```python
from build123d import *

# Parameters (mm, degrees)
F1_DEPTH      = 15
F1_DEPTH_BACK = 15
F2_R          = 1.775
F3_DEPTH      = 25
F4_W          = 5
F4_H          = 5
F5_DEPTH      = 15
F5_DEPTH_BACK = 15
F6_SIZE       = 4.99999
F7_SIZE       = 5
F8_SIZE       = 5
F9_SIZE       = 5
F10_SIZE      = 5


# Not quite as in the source:
# - a fillet or chamfer is up to 0.001 mm smaller than in the source, because OpenCascade refuses the exact size


with BuildPart() as f1:
    # F0 (on Right) → F1 (new body, two sides)
    with BuildSketch(Plane.YZ) as f1_sk:
        Polygon((-23.8343827544, 11.557416933), (-26.8343827544, 11.557416933), (-26.8343827544, -23.442583067), (8.1656172456, -23.442583067), (8.1656172456, -20.442583067), (-23.8343827544, -20.442583067), align=None)
    extrude(amount=F1_DEPTH)
    extrude(f1_sk.sketch, amount=-F1_DEPTH_BACK)

    # F2 (on face) → F3 (cut)
    with BuildSketch(Plane(origin=(0, -23.8343827544, 0), x_dir=(-1, 0, 0), z_dir=(0, 1, 0))):
        with Locations((-8.8, 5.157416933)):
            Circle(F2_R)
        with Locations((8.8, 5.157416933)):
            Circle(F2_R)
        with Locations((8.8, -8.8)):
            Circle(F2_R)
        with Locations((-8.8, -8.8)):
            Circle(F2_R)
    extrude(amount=-F3_DEPTH, mode=Mode.SUBTRACT)

    # F4 (on Right) → F5 (join, two sides)
    with BuildSketch(Plane.YZ) as f5_sk:
        with Locations((-21.3343827544, -17.942583067)):
            Rectangle(F4_W, F4_H)
    extrude(amount=F5_DEPTH)
    extrude(f5_sk.sketch, amount=-F5_DEPTH_BACK)

    # F6 (size 5 in the source; OpenCascade refuses exactly that, so slightly less here)
    f6_edges = [f1.edges().sort_by_distance(p)[0] for p in [
        (0, -18.834383, -15.442583),
    ]]
    chamfer(f6_edges, length=F6_SIZE)

    # F7
    f7_edges = [f1.edges().sort_by_distance(p)[0] for p in [
        (-15, -25.334383, 11.557417),
    ]]
    chamfer(f7_edges, length=F7_SIZE)

    # F8
    f8_edges = [f1.edges().sort_by_distance(p)[0] for p in [
        (15, -25.334383, 11.557417),
    ]]
    chamfer(f8_edges, length=F8_SIZE)

    # F9
    f9_edges = [f1.edges().sort_by_distance(p)[0] for p in [
        (15, 8.165617, -21.942583),
    ]]
    chamfer(f9_edges, length=F9_SIZE)

    # F10
    f10_edges = [f1.edges().sort_by_distance(p)[0] for p in [
        (-15, 8.165617, -21.942583),
    ]]
    chamfer(f10_edges, length=F10_SIZE)


solid = f1.part
```
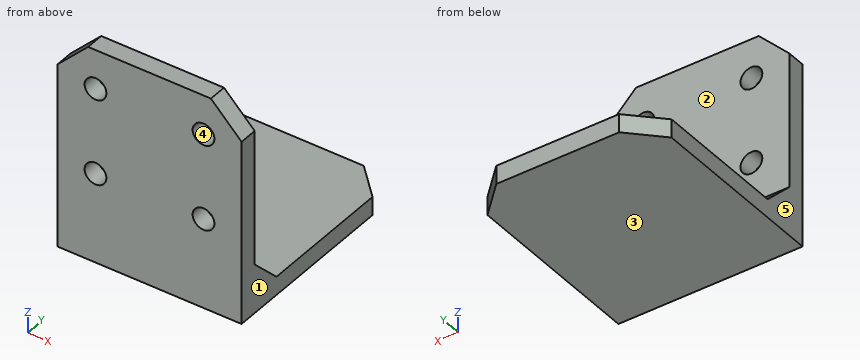
For this review, take the finished solid that the model builds, in its own axes (mm). Face numbers are marked on the shaded views. A direction names the side the tool comes from. Give positions to 0.01 mm unless a question says otherwise; leave off trailing zeros. Write each loop counter-clockwise with the first axis right and the second up, starting at its lowest first coordinate (ties: lowest second). Pieces come first, ordered by that corner, then holes.
Item 1: Take a section at D-D (y = -4.5). Give the boundary of the cut face in (x, z).
Item 2: Take a section at A-A (x = -8.8). Give the number of separate pieces and of enclosed holes in the cut face, and give its area (3 significant figures).
Item 3: Take a section at B-B (z = -8.8). Give the boundary of the cut face in (x, y) (3 decimals).
Item 4: Insertion check: P1, Ø5, axis at x = -8.5, z = -16, coming from the +Y side; P2, Ø8, axis at x = 6, z = 2.5, coming from the +Y side; P3, Ø13.5, axis at x = 5.5, y = -3.5, coming from the +Z side; P4, Ø4.5, axis at x = 8.8, z = 5.16, coming from the -Y side. Each pin has a flat end and moves straight along its axis. Give the tip position at first contact, or say it passes through.
Item 5: Wall thickness on probe 1 along Z at (x, y) = (8.8, -24.9) (3 decimals); probe 2 along X at (y, z) = (-24, -8); probe 3 along Z at (x, y) = (-8, -25): over which ranges is each line inside the solid? List them lowest first.
Item 6: The part is to be moulded in two halves that separate along Z. For the marked faces 3, 4 and 5, say which applies: +Z half, -Z half, draft (parallel to the pull), parting line (faces both ways), or undercut.
Item 7: Machinability: for the marked faces 1 and 2, which of the approach directions +Z, -Z, +X, -X, +Y, -Y give a long, thin tool a straight path to every point of the face, cutting with its end or side? Answer none if there is none.
Established:
1. outline: (-15, -23.44) - (15, -23.44) - (15, -20.44) - (-15, -20.44) - close
2. separate pieces: 3
2. enclosed holes: 0
2. area: 192 mm2
3. outline: (-15, -26.834) - (-10.575, -26.834) - (-10.575, -23.834) - (-15, -23.834) - close; (-7.025, -26.834) - (7.025, -26.834) - (7.025, -23.834) - (-7.025, -23.834) - close; (10.575, -26.834) - (15, -26.834) - (15, -23.834) - (10.575, -23.834) - close
4. P1: stops at y = -20.78
4. P2: stops at y = -23.83
4. P3: stops at z = -20.44
4. P4: stops at y = -26.83
5. probe 1: z = -23.443 to -10.575, -7.025 to 3.382, 6.932 to 11.557
5. probe 2: x = -15 to -10.38, -7.22 to 7.22, 10.38 to 15
5. probe 3: z = -23.44 to -10.38, -7.22 to 3.57, 6.74 to 11.56
6. face 3: -Z half
6. face 4: undercut
6. face 5: draft
7. face 1: +Z, -Z, +X, +Y, -Y
7. face 2: +Z, +X, -X, +Y
